The listing builds one solid part. Answer for the finished solid, in the listing's coordinates (mm). A direction names the side the tool comes from. Give positions to 0.01 mm unless a question says otherwise; leave off trailing zeros. Loops run counter-clockwise (first coordinate to the right, second up) from the corner with the lowest first, then second, coordinate; pieces in that order, holes last. Notation, with made-up numbers: M 61,-29 L 102,-29 A23 cw 102,2 Z; hole C 84,9.25 d1. An arc over 180 degrees is marked long. One line per item, written item: value. Start each with the question number.
Q1. Flat-ended cylindrical pins translate along their axes: pin 1 (3 mm diameter, centred on y = 33, z = 4, fed in from -X); pin 2 (3 mm diameter, centred on y = 13, z = 6, fed in from +X); pin 3 (1.5 mm diameter, centred on y = 30, z = 5.5, fed in from +X). Find the tip coordinate at first contact, or state that the pin passes through.
Q2. For faces 1 (the flat face through (23, 5.1, 3.9)), 2 (the cylindrical face through (44.037, 7.984, 3.944)), determine the directions among +Z, -Z, +X, -X, +Y, -Y from which every point of the face is accessible in a straight line to the end or side of a thin tool.
Q3. A cutting plane is placed at A-A, the plane z = 6.5. Determine the outline of the cut face in (x, y).
Q4. Consider L1, parallel to Y at x = 16.5, z = 7.5; L2, parallel to X at y = 22, z = 0.75; L3, parallel to Y at x = 36, z = 5.75. Determine where each line is inside the solid, lowest interval first.
Q5. The mould has two halves that part along X. Classify faces 3 (the flat face through (32, 4.701, 4)), 4 (the flat face through (21.617, 21.917, 3.944)), 5 (the cylindrical face through (29.931, 37.323, 3.944)): +X half, -X half, draft (parallel to the pull), parting line (faces both ways), or undercut.
Q6. A cutting plane is placed at C-C, the plane y = 13. Determine the outline of the cut face in (x, z).
Q7. A cutting plane is placed at B-B, the plane x = 39.5. Determine the outline of the cut face in (y, z).
from build123d import *

# Parameters (mm, degrees)
F1_DEPTH = 8
F2_R     = 3.104738


with BuildPart() as f1:
    # F0 (on Top) → F1 (new body)
    with BuildSketch(Plane.XY):
        with BuildLine():
            ThreePointArc((9.888176, 22.327356), (8.755531, 21.959757), (8.271066, 20.871958))
            Line((8.271066, 20.871958), (8.271066, 4.862583))
            ThreePointArc((8.271066, 4.862583), (8.755531, 3.774784), (9.888176, 3.407185))
            Line((9.888176, 3.407185), (20.318527, 3.407185))
            ThreePointArc((20.318527, 3.407185), (20.890308, 4.601787), (21.854779, 5.509426))
            Line((21.854779, 5.509426), (24.118731, 4.700872))
            Line((24.118731, 4.700872), (41.745216, 4.700872))
            ThreePointArc((41.745216, 4.700872), (43.721863, 7.238361), (44.494297, 10.360752))
            ThreePointArc((44.494297, 10.360752), (45.161115, 12.422565), (44.494297, 14.484379))
            ThreePointArc((44.494297, 14.484379), (46.111809, 16.465337), (44.494297, 18.446295))
            ThreePointArc((44.494297, 18.446295), (46.652767, 21.680512), (44.494297, 24.914728))
            Line((44.494297, 24.914728), (34.629937, 24.914728))
            ThreePointArc((34.629937, 24.914728), (35.295258, 31.145926), (32.770261, 36.881331))
            ThreePointArc((32.770261, 36.881331), (29.89011, 37.31441), (27.433803, 35.749357))
            Line((27.433803, 35.749357), (27.433803, 29.84691))
            Line((27.433803, 29.84691), (21.935634, 21.5188))
            Line((21.935634, 21.5188), (21.288792, 22.327356))
            Line((21.288792, 22.327356), (9.888176, 22.327356))
        make_face()
    extrude(amount=F1_DEPTH)

    # F2
    f2_edges = [f1.edges().sort_by_distance(p)[0] for p in [
        (41.745216, 4.700872, 4),
    ]]
    fillet(f2_edges, radius=F2_R)


solid = f1.part
Answer block:
1. pin 1: x = 27.43
1. pin 2: x = 45.16
1. pin 3: x = 35.44
2. face 1: +Z, -Z, -Y
2. face 2: +Z, -Z, +X, -Y
3. outline: M 8.27,4.86 A1.46 ccw 9.89,3.41 L 20.32,3.41 A3.61 cw 21.85,5.51 L 24.12,4.7 L 40.44,4.7 A3.1 ccw 42.91,5.92 A7.73 ccw 44.49,10.36 A3.52 ccw 44.49,14.48 A2.02 ccw 44.49,18.45 A3.5 ccw 44.49,24.91 L 34.63,24.91 A12.16 ccw 32.77,36.88 A4.15 ccw 27.43,35.75 L 27.43,29.85 L 21.94,21.52 L 21.29,22.33 L 9.89,22.33 A1.46 ccw 8.27,20.87 Z
4. L1: 3.41 to 22.33
4. L2: 8.8 to 21.55, 22.25 to 46.64
4. L3: 4.7 to 24.91
5. face 3: draft
5. face 4: undercut
5. face 5: parting line
6. outline: M 8.27,0 L 45.11,0 L 45.11,8 L 8.27,8 Z
7. outline: M 4.7,0 L 24.91,0 L 24.91,8 L 4.7,8 Z
